The listing builds one solid part. Answer for the finished solid, in the listing's coordinates (mm). A direction names the side the tool comes from. Round coordinates to 2 decimals unless told otherwise and drop trailing zeros. Write each loop counter-clockwise with the first axis right and the second up, starting at its lowest first coordinate (ties: lowest second). Pieces come first, ordered by that corner, then holes.
from build123d import *

# Parameters (mm, degrees)
F0_W     = 18
F0_H     = 23
F1_DEPTH = 16
F2_R     = 0.75
F8_R     = 2


with BuildPart() as f1:
    # F0 (on Top) → F1 (new body)
    with BuildSketch(Plane.XY):
        with Locations((9, 11.5)):
            Rectangle(F0_W, F0_H)
    extrude(amount=F1_DEPTH)

    # F5: sweep along a path in F4
    with BuildLine(Plane(origin=(2, 0, 0), x_dir=(0, -1, 0), z_dir=(-1, 0, 0))) as f5_path:
        add(Plane(origin=(2, 0, 0), x_dir=(0, -1, 0), z_dir=(-1, 0, 0)) * Edge.make_bspline(
            [(-23.0005215853, 3.1891802792), (-23.7749723998, 3.0223947387), (-25.4927262434, 2.6524596858), (-26.7959816722, 6.2629262385), (-32.8904530092, 6.2095022364), (-33.6051186574, 6.259200929), (-33.8062010705, 6.2731844373)],
            knots=[0, 0, 0, 0, 0.2232557328, 0.4951875392, 0.8579630796, 1, 1, 1, 1], degree=3))
    # F2 (on face) → F5 (sweep)
    with BuildSketch(Plane(origin=(0, 23, 0), x_dir=(-1, 0, 0), z_dir=(0, 1, 0))):
        with Locations((-2, 3.1886692159)):
            Circle(F2_R)
    sweep(path=f5_path.line)

    # F7: F1 across plane


with BuildPart() as f1_1:
    add(f1.part)
    add(f1.part.mirror(Plane(origin=(9, 11.5, 8), x_dir=(1, 0, 0), z_dir=(0, 0, -1))))

    # F8
    f8_edges = [f1_1.edges().sort_by_distance(p)[0] for p in [
        (0, 11.5, 16),
        (0, 11.5, 0),
        (18, 11.5, 0),
        (18, 0, 8),
        (9, 0, 0),
        (9, 0, 16),
        (0, 0, 8),
        (9, 23, 16),
        (18, 23, 8),
        (9, 23, 0),
        (18, 11.5, 16),
    ]]
    fillet(f8_edges, radius=F8_R)


solid = f1_1.part
1. For a pull along Z with two mould halves and no side action, classify faces 3 (the face through (2.038, 33.808, 9.734)), 4 (the face through (8.11, 22.43, 0.6)), 5 (the face through (9, 0, 8)) as released by +Z, released by -Z, zero draft, split by the parting line, or undercut.
Geometry says:
face 3: undercut
face 4: released by -Z
face 5: zero draft
2. Straight lines are drawn through the part: line 1 along Y through (x, z) = (4.5, 5); line 2 along Y through (x, z) = (2.5, 11.5); line 3 along Z through (x, y) = (2.75, 22.5). For each, find the intervals that lie inside material, in ascending order.
Geometry says:
line 1: y = 0 to 23
line 2: y = 0 to 23, 25.64 to 27.11
line 3: z = 0.68 to 15.32
3. Section A-A on x = 4.25 is taken. Determine the outline of the cut face in (y, z).
Geometry says:
outline: (0, 2) arc R2 ccw to (2, 0) - (21, 0) arc R2 ccw to (23, 2) - (23, 14) arc R2 ccw to (21, 16) - (2, 16) arc R2 ccw to (0, 14) - close
4. Given pin 1 (3 mm diameter, centred on x = 4.5, z = 4.5, fed in from +Y); pin 2 (5 mm diameter, centred on y = 27, z = 9.5, fed in from +X), each flat-ended and moving along its own axis, determine where each tip first touches the part or whether it passes through.
Geometry says:
pin 1: stops at y = 23
pin 2: stops at x = 2.75
5. A tool of negligible diameter and unlimited length cuts with its end or side. For faces 1 (the face through (9.1, 0.57, 15.4)), 2 (the face through (2.038, 33.808, 6.266)), from which of +Z, -Z, +X, -X, +Y, -Y can it reach the whole face along a straight path? Write none if from no direction.
Geometry says:
face 1: +Z, +X, -X, -Y
face 2: +X, -X, +Y
6. Section C-C on x = 16.5 is taken. Determine the outline of the cut face in (y, z), plus the area to 3 significant figures.
Geometry says:
outline: (0.06, 2) arc R1.94 ccw to (2, 0.06) - (21, 0.06) arc R1.94 ccw to (22.94, 2) - (22.94, 14) arc R1.94 ccw to (21, 15.94) - (2, 15.94) arc R1.94 ccw to (0.06, 14) - close
area: 360 mm2
7. Section B-B on z = 1 is taken. Determine the outline of the cut face in (x, y).
Geometry says:
outline: (0.27, 2) arc R1.73 ccw to (2, 0.27) - (16, 0.27) arc R1.73 ccw to (17.73, 2) - (17.73, 21) arc R1.73 ccw to (16, 22.73) - (0.27, 22.73) - close
